from build123d import *

# Parameters (mm, degrees)
BOSS_EXTRUDE1_DEPTH = 177.8
SKETCH2_W           = 12.7
SKETCH2_H           = 2.54
BOSS_EXTRUDE2_DEPTH = 177.8
SKETCH3_R           = 3.175
CUT_EXTRUDE1_DEPTH  = 203.727168628
SKETCH4_W           = 31.75
SKETCH4_H           = 6.35
BOSS_EXTRUDE3_DEPTH = 152.4
FILLET1_R           = 2.54
BOSS_EXTRUDE4_REACH = 251.919
SKETCH5_W           = 31.75
SKETCH5_H           = 6.35
BOSS_EXTRUDE5_DEPTH = 6.35
SKETCH7_W           = 25.4
SKETCH7_H           = 6.35
BOSS_EXTRUDE6_DEPTH = 12.7
SKETCH8_W           = 12.7
SKETCH8_H           = 6.35
REVOLVE1_ANGLE      = 180
SKETCH10_R          = 6.35
CUT_EXTRUDE2_DEPTH  = 206.273019416
SKETCH11_R          = 12.7
BOSS_EXTRUDE7_DEPTH = 457.2
BOSS_EXTRUDE8_DEPTH = 2.54
CUT_EXTRUDE3_DEPTH  = 646.740988406


with BuildPart() as part:
    # Sketch1 → Boss-Extrude1 (new body)
    with BuildSketch(Plane(origin=(0, 0, 0), x_dir=(1, 0, 0), z_dir=(0, 1, 0))):
        Polygon((76.2, 0), (82.55, 0), (82.55, 38.1), (-82.55, 38.1), (-82.55, 0), (-76.2, 0), (-76.2, 31.75), (76.2, 31.75), align=None)
    extrude(amount=BOSS_EXTRUDE1_DEPTH)

    # Sketch2 → Boss-Extrude2 (add)
    with BuildSketch(Plane(origin=(0, 177.8, 0), x_dir=(1, 0, 0), z_dir=(0, 1, 0))):
        with Locations((88.9, 30.48)):
            Rectangle(SKETCH2_W, SKETCH2_H)
        with Locations((88.9, 21.59)):
            Rectangle(SKETCH2_W, SKETCH2_H)
        with Locations((-88.9, 21.59)):
            Rectangle(SKETCH2_W, SKETCH2_H)
        with Locations((-88.9, 30.48)):
            Rectangle(SKETCH2_W, SKETCH2_H)
    extrude(amount=-BOSS_EXTRUDE2_DEPTH)

    # Sketch3 → Cut-Extrude1 (cut, through all)
    with BuildSketch(Plane.XY.offset(-20.32)):
        with Locations((88.9, 12.7)):
            Circle(SKETCH3_R)
        with Locations((88.9, 88.9)):
            Circle(SKETCH3_R)
        with Locations((88.9, 165.1)):
            Circle(SKETCH3_R)
        with Locations((-88.9, 12.7)):
            Circle(SKETCH3_R)
        with Locations((-88.9, 165.1)):
            Circle(SKETCH3_R)
        with Locations((-88.9, 88.9)):
            Circle(SKETCH3_R)
    extrude(amount=-CUT_EXTRUDE1_DEPTH, mode=Mode.SUBTRACT)

    # Sketch4 → Boss-Extrude3 (add)
    with BuildSketch(Plane(origin=(-76.2, 0, 0), x_dir=(0, 0, -1), z_dir=(1, 0, 0))):
        with Locations((15.875, 3.175)):
            Rectangle(SKETCH4_W, SKETCH4_H)
    extrude(amount=BOSS_EXTRUDE3_DEPTH)

    # Fillet1
    fillet1_edges = [part.edges().sort_by_distance(p)[0] for p in [
        (76.2, 6.35, -15.875),
        (0, 6.35, -31.75),
        (-76.2, 6.35, -15.875),
    ]]
    fillet(fillet1_edges, radius=FILLET1_R)

    # Sketch5 → Boss-Extrude4 (add, up to next)
    with BuildSketch(Plane(origin=(-76.2, 0, 0), x_dir=(0, 0, -1), z_dir=(1, 0, 0)), mode=Mode.PRIVATE) as boss_extrude4_sk1:
        with Locations((15.875, 174.625)):
            Rectangle(SKETCH5_W, SKETCH5_H)
    boss_extrude4_tool1 = extrude(boss_extrude4_sk1.sketch, amount=BOSS_EXTRUDE4_REACH, mode=Mode.PRIVATE) - part.part
    add(boss_extrude4_tool1.solids().sort_by_distance((-76.2, 174.625, -15.875))[0])

    # Sketch6 → Boss-Extrude5 (add)
    with BuildSketch(Plane.XY):
        with BuildLine():
            Line((76.2, 171.45), (76.2, 8.89))
            ThreePointArc((76.2, 8.89), (75.456051224, 7.093948776), (73.66, 6.35))
            Line((73.66, 6.35), (-73.66, 6.35))
            ThreePointArc((-73.66, 6.35), (-75.456051224, 7.093948776), (-76.2, 8.89))
            Line((-76.2, 8.89), (-76.2, 171.45))
            Line((-76.2, 171.45), (76.2, 171.45))
        make_face()
    extrude(amount=-BOSS_EXTRUDE5_DEPTH)

    # Sketch7 → Boss-Extrude6 (add)
    with BuildSketch(Plane.XZ):
        with Locations((0, -3.175)):
            Rectangle(SKETCH7_W, SKETCH7_H)
        with Locations((0, -34.925)):
            Rectangle(SKETCH7_W, SKETCH7_H)
    extrude(amount=BOSS_EXTRUDE6_DEPTH)

    # Sketch8 → Revolve1 (revolve)
    with BuildSketch(Plane.XZ.offset(12.7)):
        with Locations((6.35, -3.175)):
            Rectangle(SKETCH8_W, SKETCH8_H)
        with Locations((6.35, -34.925)):
            Rectangle(SKETCH8_W, SKETCH8_H)
    revolve(axis=Axis((0, -12.7, 0), (0, 0, -1)), revolution_arc=REVOLVE1_ANGLE)

    # Sketch10 → Cut-Extrude2 (cut, through all)
    with BuildSketch(Plane(origin=(0, 0, -38.1), x_dir=(-1, 0, 0), z_dir=(0, 0, -1))):
        with Locations((0, -12.7)):
            Circle(SKETCH10_R)
    cut_extrude2 = extrude(amount=-CUT_EXTRUDE2_DEPTH, mode=Mode.SUBTRACT)

    # Sketch11 → Boss-Extrude7 (add)
    with BuildSketch(Plane(origin=(0, 177.8, 0), x_dir=(1, 0, 0), z_dir=(0, 1, 0))):
        with Locations(Location((-41.275, 19.05, 0), (0, 0, 90))):
            Circle(SKETCH11_R)
        with Locations(Location((41.275, 19.05, 0), (0, 0, 90))):
            Circle(SKETCH11_R)
    extrude(amount=BOSS_EXTRUDE7_DEPTH)

    # Sketch12 → Boss-Extrude8 (add)
    with BuildSketch(Plane(origin=(0, 635, 0), x_dir=(1, 0, 0), z_dir=(0, 1, 0))):
        Polygon((82.55, 0), (82.55, 20.32), (82.55, 22.86), (82.55, 29.21), (82.55, 31.75), (82.55, 38.1), (-82.55, 38.1), (-82.55, 31.75), (-82.55, 29.21), (-82.55, 22.86), (-82.55, 20.32), (-82.55, 0), align=None)
    extrude(amount=BOSS_EXTRUDE8_DEPTH)

    # Mirror1: Cut-Extrude2 across plane
    add(cut_extrude2.mirror(Plane.ZX), mode=Mode.SUBTRACT)

    # Sketch13 → Cut-Extrude3 (cut, through all)
    with BuildSketch(Plane.XY):
        with BuildLine():
            Line((-12.7, 0), (12.7, 0))
            Line((12.7, 0), (12.7, -12.7))
            ThreePointArc((12.7, -12.7), (0, -25.4), (-12.7, -12.7))
            Line((-12.7, -12.7), (-12.7, 0))
        make_face()
    extrude(amount=-CUT_EXTRUDE3_DEPTH, mode=Mode.SUBTRACT)


solid = part.part
Work out the finished part from the listing and answer in its coordinate system (mm). A direction names the side the tool comes from. Round coordinates to 2 decimals unless told otherwise and drop trailing zeros. Write each loop counter-clockwise with the first axis right and the second up, starting at its lowest first coordinate (ties: lowest second). Pieces come first, ordered by that corner, then holes.
1) A cutting plane is placed at A-A (x = -21). Give the vertices of the cut face in (y, z), plus the area to 3 significant figures.
2) Straight lines are drawn through the part: line 1 (Y direction, x = -55, z = -14.5); line 2 (Y direction, x = -88, z = -31); line 3 (X direction, y = 165, z = -21). For each, find the intervals that lie inside material, in ascending order.
3) Given pin 1 Ø4 at (y, z) = (125, -4) entering from +X; pin 2 Ø5 at (y, z) = (85, -25.5) entering from -X; pin 3 Ø6.5 at (x, y) = (-86.5, 51.5) entering from +Z, each flat-ended and moving along its own axis, determine where each tip first touches the part or whether it passes through.
4) A tool of negligible diameter and unlimited length cuts with its end or side. For faces 4 (the flat face through (-93, 90, -22.86)), 5 (the flat face through (85, 90, -31.75)), 6 (the cylindrical face through (-30.01, 403.2, -24.91)), 7 (the flat face through (-93, 90, -31.75)), from which of +Z, -Z, +X, -X, +Y, -Y can it reach the whole face along a straight path? Write none if from no direction.
5) A cutting plane is placed at B-B (y = 271). Give the vertices of the cut face in (x, z) (3 decimals).
6) The mould has two halves that part along X. Classify faces 1 (the flat face through (1, 88, 0)), 2 (the flat face through (82.55, 88, -10)), 3 (the flat face through (-1, 89, -31.75)): pulls with the +X half, pulls with the -X half, needs draft (parallel to the pull), parting line crosses it, or undercut.
Completed:
1. outline: (0, -38.1) - (177.8, -38.1) - (177.8, 0) - (0, 0) - close; (635, -38.1) - (637.54, -38.1) - (637.54, 0) - (635, 0) - close; hole (6.35, -29.21) arc R2.54 ccw to (8.89, -31.75) - (171.45, -31.75) - (171.45, -6.35) - (6.35, -6.35) - close
1. area: 2,680 mm2
2. line 1: y = 0 to 6.35, 171.45 to 177.8, 635 to 637.54
2. line 2: y = 0 to 9.66, 15.74 to 85.86, 91.94 to 162.06, 168.14 to 177.8
2. line 3: x = -95.25 to -92.07, -85.73 to -76.2, 76.2 to 85.73, 92.07 to 95.25
3. pin 1: stops at x = 82.55
3. pin 2: stops at x = -82.55
3. pin 3: stops at z = -20.32
4. face 4: -X, +Y, -Y
4. face 5: -Z, +X, +Y, -Y
4. face 6: none
4. face 7: -Z, -X, +Y, -Y
5. outline: circle Ø25.4 at (-41.275, -19.05); circle Ø25.4 at (41.275, -19.05)
6. face 1: needs draft
6. face 2: pulls with the +X half
6. face 3: undercut
